from build123d import *

# Parameters (mm, degrees)
SKETCH1_W           = 110
SKETCH1_H           = 40
BOSS_EXTRUDE1_DEPTH = 3
BOSS_EXTRUDE2_DEPTH = 3
SKETCH3_R           = 1
CUT_EXTRUDE1_DEPTH  = 3
SKETCH4_W           = 8
SKETCH4_H           = 3
SKETCH4_W_2         = 2.4
SKETCH4_H_2         = 6
CUT_EXTRUDE2_DEPTH  = 3
FILLET6_R           = 1
SKETCH6_R           = 1.25
CUT_EXTRUDE4_DEPTH  = 62.424750712


with BuildPart() as part:
    # Sketch1 → Boss-Extrude1 (new body)
    with BuildSketch(Plane.XY):
        Rectangle(SKETCH1_W, SKETCH1_H)
    extrude(amount=BOSS_EXTRUDE1_DEPTH)

    # Sketch2 → Boss-Extrude2 (add)
    with BuildSketch(Plane.XY.offset(3)):
        Polygon((58, 10), (58, 13.5), (55, 13.5), (55, 6.5), (58, 6.5), align=None)
        Polygon((55, -10), (55, -6.5), (58, -6.5), (58, -13.5), (55, -13.5), align=None)
        Polygon((-55, 6.5), (-55, 13.5), (-58, 13.5), (-58, 10), (-58, 6.5), align=None)
        Polygon((-55, -13.5), (-55, -10), (-55, -6.5), (-58, -6.5), (-58, -13.5), align=None)
    extrude(amount=-BOSS_EXTRUDE2_DEPTH)

    # Sketch3 → Cut-Extrude1 (cut)
    with BuildSketch(Plane.XY.offset(3)):
        with Locations((-55, 14.5)):
            Circle(SKETCH3_R)
        with Locations((-55, 5.5)):
            Circle(SKETCH3_R)
        with Locations((-55, -5.5)):
            Circle(SKETCH3_R)
        with Locations((-55, -14.5)):
            Circle(SKETCH3_R)
        with Locations((55, 14.5)):
            Circle(SKETCH3_R)
        with Locations((55, 5.5)):
            Circle(SKETCH3_R)
        with Locations((55, -5.5)):
            Circle(SKETCH3_R)
        with Locations((55, -14.5)):
            Circle(SKETCH3_R)
    extrude(amount=-CUT_EXTRUDE1_DEPTH, mode=Mode.SUBTRACT)

    # Sketch4 → Cut-Extrude2 (cut)
    with BuildSketch(Plane.XY.offset(3)):
        with Locations((-51, 0)):
            Rectangle(SKETCH4_W, SKETCH4_H)
        Polygon((-47, 3), (-47, 1.5), (-47, -1.5), (-47, -3), (-44.6, -3), (-44.6, -1.5), (-44.6, 1.5), (-44.6, 3), align=None)
        with BuildLine():
            ThreePointArc((-44.6, -1.5), (-43.1, 0), (-44.6, 1.5))
            Line((-44.6, 1.5), (-44.6, -1.5))
        make_face()
        with Locations((45.8, 0)):
            Rectangle(SKETCH4_W_2, SKETCH4_H_2)
        with BuildLine():
            Line((44.6, -1.5), (44.6, 1.5))
            ThreePointArc((44.6, 1.5), (43.1, 0), (44.6, -1.5))
        make_face()
        with Locations((51, 0)):
            Rectangle(SKETCH4_W, SKETCH4_H)
    extrude(amount=-CUT_EXTRUDE2_DEPTH, mode=Mode.SUBTRACT)

    # Fillet6
    fillet6_edges = [part.edges().sort_by_distance(p)[0] for p in [
        (-47, 3, 1.5),
        (-44.6, 3, 1.5),
        (-44.6, -3, 1.5),
        (-47, -3, 1.5),
        (47, 3, 1.5),
        (47, -3, 1.5),
        (44.6, -3, 1.5),
        (44.6, 3, 1.5),
    ]]
    fillet(fillet6_edges, radius=FILLET6_R)

    # Sketch6 → Cut-Extrude4 (cut, through all)
    with BuildSketch(Plane.XY.offset(3)):
        with Locations((-40, -14)):
            Circle(SKETCH6_R)
        with Locations((-20, -14)):
            Circle(SKETCH6_R)
        with Locations((0, -14)):
            Circle(SKETCH6_R)
        with Locations((20, -14)):
            Circle(SKETCH6_R)
        with Locations((40, -14)):
            Circle(SKETCH6_R)
        with Locations((40, 14)):
            Circle(SKETCH6_R)
        with Locations((20, 14)):
            Circle(SKETCH6_R)
        with Locations((0, 14)):
            Circle(SKETCH6_R)
        with Locations((-20, 14)):
            Circle(SKETCH6_R)
        with Locations((-40, 14)):
            Circle(SKETCH6_R)
    extrude(amount=-CUT_EXTRUDE4_DEPTH, mode=Mode.SUBTRACT)


solid = part.part
Could you check a few things on this model? Use its own coordinates, in mm. A direction names the side the tool comes from. Coordinates: 2 decimals unless noted, no trailing zeros. Order: outer loops, then holes, each group sorted by start corner. A loop starts at its lowest first (then second) coordinate and runs counter-clockwise, first axis right, second up. Notation, with made-up numbers: (-18, 20) - (24, 20) arc R22 ccw to (24, 45) - close; hole circle Ø3 at (80.5, 1). An arc over 180 degrees is marked (long way). Answer in a Markdown table with one row per item. Add a question column.
(1) If we section it at B-B, the plane z = 2.45: State how many separate pieces and enclosed holes the cut face has, then the cut area to 3 significant figures.
(2) I need wall thicknesses on L1, parallel to Y at x = -20, z = 1.8; L2, parallel to Y at x = 48.5, z = 2.55; L3, parallel to X at y = -3.5, z = 0.4. Which ranges of each line are inside material? Lowest first, please.
(3) If we section it at A-A, the plane x = 0: Please give me the cut outline in (y, z), then the cut area to 3 significant figures.
(4) If we section it at D-D, the plane y = -5.5: Please give me the cut outline in (x, z).
(5) Will these pins go through, and if not, where does the flat tip stop? pin 1 (0.6 mm diameter, centred on y = -1.5, z = 1, fed in from -X); pin 2 (0.9 mm diameter, centred on x = 57, z = 1.5, fed in from -Y); pin 3 (0.9 mm diameter, centred on y = -17, z = 1.5, fed in from +X); pin 4 (2 mm diameter, centred on x = 0, y = 14, fed in from +Z).
(6) On a 3-axis mill with a long thin cutter (end or side, diameter ignored), from which of +Z, -Z, +X, -X, +Y, -Y can I reach the whole of each face in a straight line? I mean faces 1 (the face through (-51, -1.5, 2)), 2 (the face through (55, -18, 1)), 3 (the face through (55, 3, 1)). Say none if no direction works.
(7) If we mould it in two halves opening along Y, with no side actions, what happens to faces 4 (the face through (-56, 13.5, 2)), 5 (the face through (58, 10, 2)), 6 (the face through (-51, 1.5, 2))? For each: released by +Y, released by -Y, zero draft, split by the parting line, or undercut.
(8) If we section it at C-C, the plane y = -17: Please give me the cut outline in (x, z).
Results are:
| question | item | result |
|---|---|---|
| 1 | separate pieces | 1 |
| 1 | enclosed holes | 10 |
| 1 | area | 4,340 mm2 |
| 2 | L1 | y = -20 to -15.25, -12.75 to 12.75, 15.25 to 20 |
| 2 | L2 | y = -20 to -1.5, 1.5 to 20 |
| 2 | L3 | x = -55 to 55 |
| 3 | outline | (-20, 0) - (-15.25, 0) - (-15.25, 3) - (-20, 3) - close; (-12.75, 0) - (12.75, 0) - (12.75, 3) - (-12.75, 3) - close; (15.25, 0) - (20, 0) - (20, 3) - (15.25, 3) - close |
| 3 | area | 105 mm2 |
| 4 | outline | (-54, 0) - (54, 0) - (54, 3) - (-54, 3) - close |
| 5 | pin 1 | stops at x = -55 |
| 5 | pin 2 | stops at y = -13.5 |
| 5 | pin 3 | stops at x = 55 |
| 5 | pin 4 | passes through |
| 6 | face 1 | +Z, -Z, -X |
| 6 | face 2 | +Z, -Z, +X, -Y |
| 6 | face 3 | +Z, -Z, +X |
| 7 | face 4 | released by +Y |
| 7 | face 5 | zero draft |
| 7 | face 6 | undercut |
| 8 | outline | (-55, 0) - (55, 0) - (55, 3) - (-55, 3) - close |
